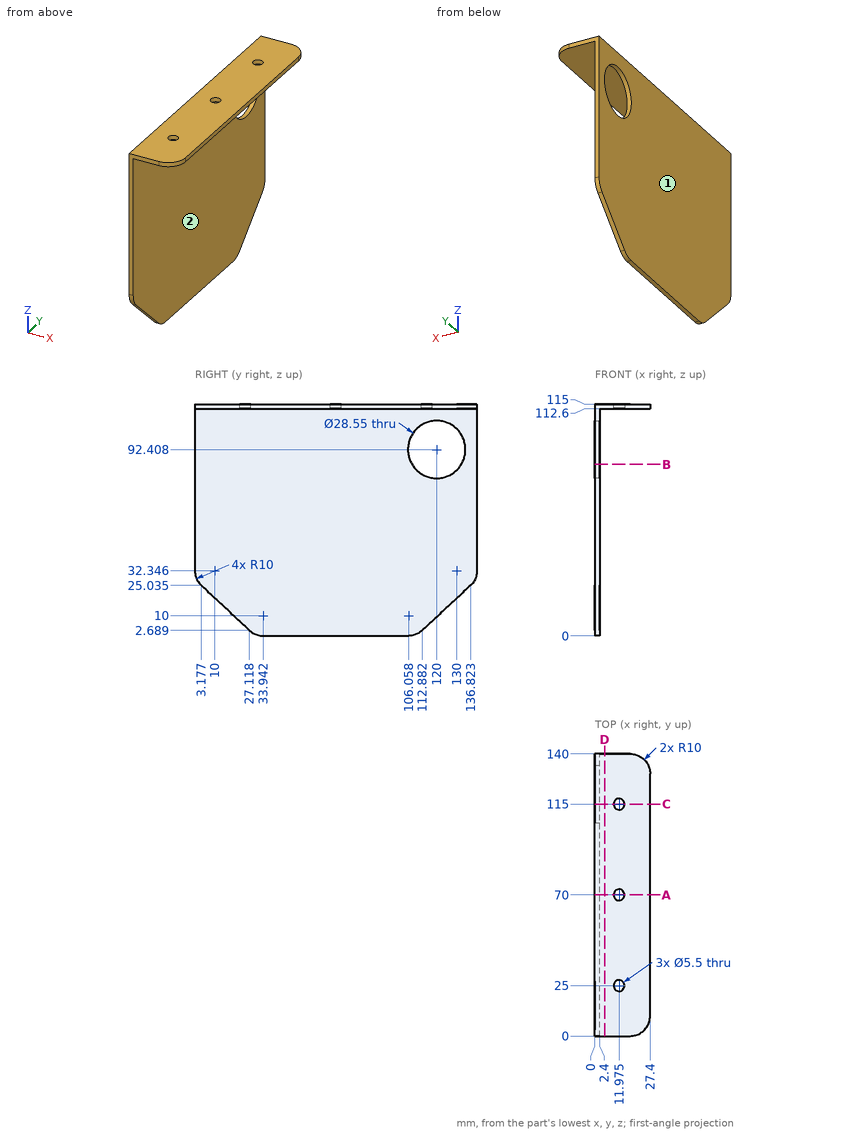
Study the drawing (mm; zero at the part's minimum x, y, z) and answer. A direction names the side the tool comes from. Give positions to 0.01 mm unless a question says otherwise; leave off trailing zeros. Write each loop counter-clockwise with the first axis right and the second up, starting at its lowest first coordinate (ties: lowest second). Pieces come first, ordered by that corner, then holes. Notation, with made-up numbers: M -9.75,80 L 48.25,80 A29 cw 48.25,107 Z; hole C -39,54.5 d1. An arc over 180 degrees is marked long. Put each result on its own line as item: value. Start each with the question number.
1. The part is cut by section C-C, the plane y = 115. Give the vertices of the cut face in (x, z) (1 decimal).
2. Each of these flat-tipped pins is pushed along its axis until it touches: pin 1 Ø1.5 at (y, z) = (103, 90) entering from +X; pin 2 Ø8 at (x, y) = (16.5, 100.5) entering from -Z; pin 3 Ø5 at (x, y) = (11.97, 115) entering from +Z. Where does it stop, or does it pass through?
3. The part is cut by section D-D, the plane x = 4.75. Give the vertices of the cut face in (y, z), and give its area (3 significant figures).
4. Which of the six approach directions +Z, -Z, +X, -X, +Y, -Y give full straight-line access (tool end or side, diameter ignored) to the marked faces 1 and 2?
5. The part is cut by section B-B, the plane z = 85. Give the vertices of the cut face in (x, y).
6. The part is cut by section A-A, the plane y = 70. Give the vertices of the cut face in (x, z) (1 decimal), and give its area (3 significant figures).
7. Consider line 1 along X through (y, z) = (115, 113.6) (1 decimal); line 2 along X through (y, z) = (10, 86); line 3 along Z through (x, y) = (2.25, 122.5) (1 decimal). Determine where each line is inside the solid, lowest interval first.
Final values:
1. outline: M 0,4.7 L 2.4,4.7 L 2.4,79 L 0,79 Z; M 0,105.8 L 2.4,105.8 L 2.4,112.6 L 9.2,112.6 L 9.2,115 L 0,115 Z; M 14.7,112.6 L 27.4,112.6 L 27.4,115 L 14.7,115 Z
2. pin 1: stops at x = 2.4
2. pin 2: stops at z = 112.6
2. pin 3: passes through
3. outline: M 0,112.6 L 140,112.6 L 140,115 L 0,115 Z
3. area: 336 mm²
4. face 1: +Z, -Z, -X, +Y, -Y
4. face 2: -Z, +X, +Y, -Y
5. outline: M 0,0 L 2.4,0 L 2.4,107.8 L 0,107.8 Z; M 0,132.2 L 2.4,132.2 L 2.4,140 L 0,140 Z
6. outline: M 0,0 L 2.4,0 L 2.4,112.6 L 9.2,112.6 L 9.2,115 L 0,115 Z; M 14.7,112.6 L 27.4,112.6 L 27.4,115 L 14.7,115 Z
6. area: 323 mm²
7. line 1: x = 0 to 9.2, 14.7 to 27.4
7. line 2: x = 0 to 2.4
7. line 3: z = 11.7 to 78.4, 106.5 to 115
